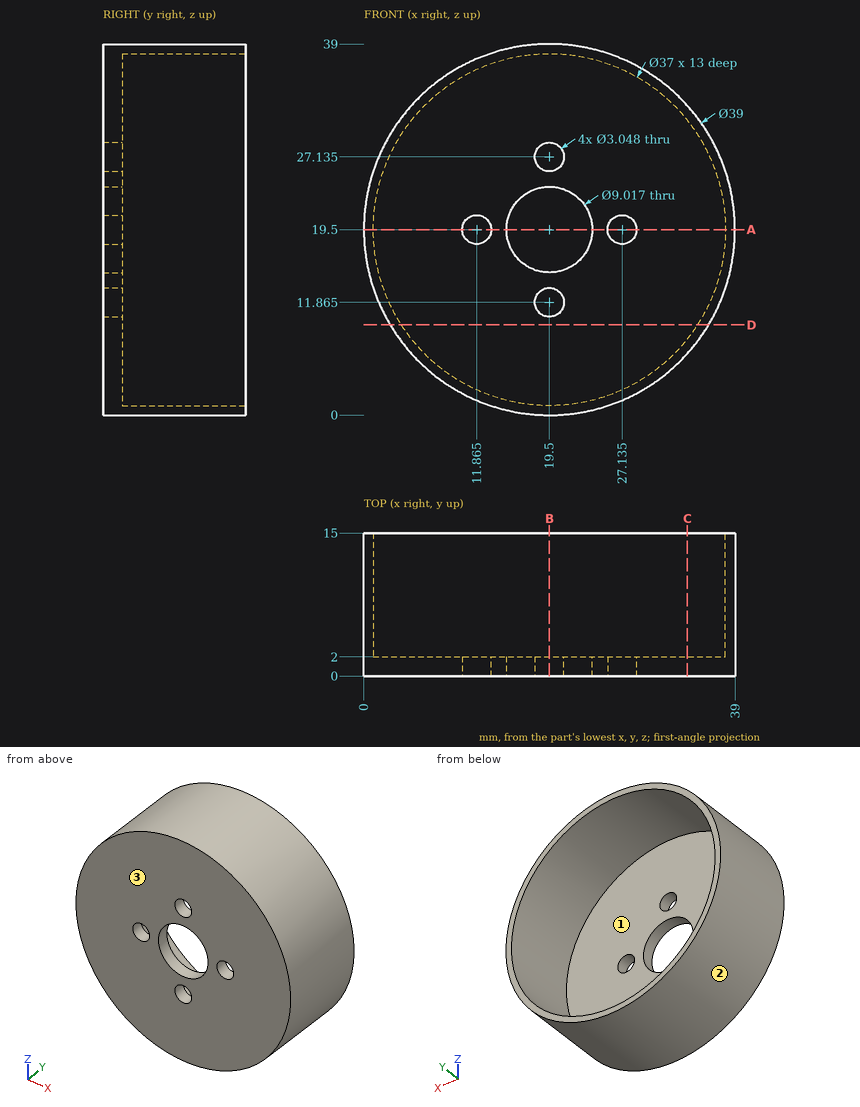
Geometry check sheet. Reference: drawing and pictorial views, mm from the part's lowest x, y, z. Coordinates: 2 decimals unless noted, no trailing zeros. Loops run counter-clockwise (first coordinate to the right, second up) from the corner with the lowest first, then second, coordinate; pieces in that order, holes last.
1) Sectioned sample at B-B (x = 19.5). Record the boundary of the cut face in (y, z).
2) Sectioned sample at C-C (x = 34). Record the boundary of the cut face in (y, z).
3) Sectioned sample at A-A (z = 19.5). Record the boundary of the cut face in (x, y).
4) Gauge pin test, flat ends, axial feed: pin 1 (1 mm diameter, centred on x = 21.5, y = 5.5, fed in from -Z); pin 2 (3 mm diameter, centred on y = 4, z = 29.5, fed in from -X); pin 3 (2.5 mm diameter, centred on x = 11.86, z = 19.5, fed in from -Y); pin 4 (1.5 mm diameter, centred on x = 31, y = 12, fed in from -Z). Record the tip position at first contact, or that the pin passes through.
5) Sectioned sample at D-D (z = 9.5). Record the boundary of the cut face in (x, y).
6) Material ranges on probe 1 along Z at (x, y) = (19.5, 0.75); probe 2 along Z at (x, y) = (19.5, 7.25); probe 3 along Y at (x, z) = (19, 31), recorded low to high.
7) Release check for a two-part mould opening along Z. For the marked faces 1, 2 and 3 record: released by +Z, released by -Z, zero draft, split by the parting line, or undercut.
Check sheet entries:
1. outline: (0, 0) - (15, 0) - (15, 1) - (2, 1) - (2, 10.34) - (0, 10.34) - close; (0, 13.39) - (2, 13.39) - (2, 14.99) - (0, 14.99) - close; (0, 24.01) - (2, 24.01) - (2, 25.61) - (0, 25.61) - close; (0, 28.66) - (2, 28.66) - (2, 38) - (15, 38) - (15, 39) - (0, 39) - close
2. outline: (0, 6.46) - (15, 6.46) - (15, 8.01) - (2, 8.01) - (2, 30.99) - (15, 30.99) - (15, 32.54) - (0, 32.54) - close
3. outline: (0, 0) - (10.34, 0) - (10.34, 2) - (1, 2) - (1, 15) - (0, 15) - close; (13.39, 0) - (14.99, 0) - (14.99, 2) - (13.39, 2) - close; (24.01, 0) - (25.61, 0) - (25.61, 2) - (24.01, 2) - close; (28.66, 0) - (39, 0) - (39, 15) - (38, 15) - (38, 2) - (28.66, 2) - close
4. pin 1: stops at z = 0.06
4. pin 2: stops at x = 1.95
4. pin 3: passes through
4. pin 4: stops at z = 3.23
5. outline: (2.76, 0) - (36.24, 0) - (36.24, 15) - (35.06, 15) - (35.06, 2) - (3.94, 2) - (3.94, 15) - (2.76, 15) - close
6. probe 1: z = 0 to 10.34, 13.39 to 14.99, 24.01 to 25.61, 28.66 to 39
6. probe 2: z = 0 to 1, 38 to 39
6. probe 3: y = 0 to 2
7. face 1: undercut
7. face 2: split by the parting line
7. face 3: zero draft
